```python
from build123d import *

# Parameters (mm, degrees)
BOSS_EXTRUDE1_DEPTH = 6.35
SKETCH2_W           = 25
SKETCH2_H           = 18.64
CUT_EXTRUDE1_DEPTH  = 91.434078201


with BuildPart() as part:
    # Sketch1 → Boss-Extrude1 (new body)
    with BuildSketch(Plane(origin=(0, 0, 0), x_dir=(1, 0, 0), z_dir=(0, 1, 0))):
        with BuildLine():
            Line((7, 0), (70, 0))
            ThreePointArc((70, 0), (74.949747468, 2.050252532), (77, 7))
            Line((77, 7), (77, 40))
            ThreePointArc((77, 40), (74.949747468, 44.949747468), (70, 47))
            Line((70, 47), (7, 47))
            ThreePointArc((7, 47), (2.050252532, 44.949747468), (0, 40))
            Line((0, 40), (0, 7))
            ThreePointArc((0, 7), (2.050252532, 2.050252532), (7, 0))
        make_face()
    extrude(amount=BOSS_EXTRUDE1_DEPTH)

    # Sketch2 → Cut-Extrude1 (cut, through all)
    with BuildSketch(Plane(origin=(0, 6.35, 0), x_dir=(1, 0, 0), z_dir=(0, 1, 0))):
        with Locations((38.5, 16.32)):
            Rectangle(SKETCH2_W, SKETCH2_H)
    extrude(amount=-CUT_EXTRUDE1_DEPTH, mode=Mode.SUBTRACT)


solid = part.part
```
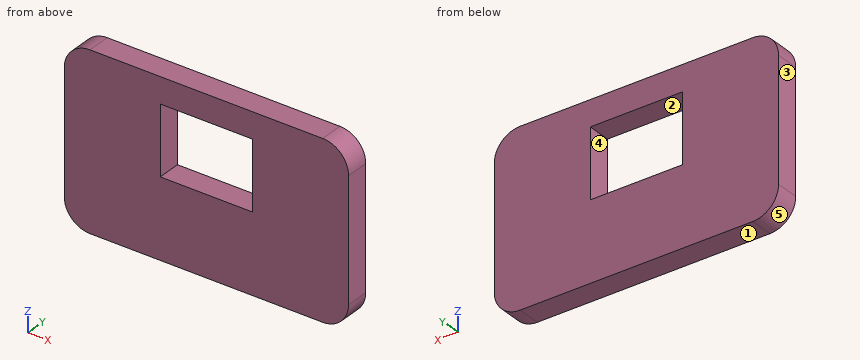
The listing builds one solid part. Answer for the finished solid, in the listing's coordinates (mm). Face numbers are marked on the shaded views. A direction names the side the tool comes from. Give positions to 0.01 mm unless a question says otherwise; leave off trailing zeros. Order: outer loops, then holes, each group sorted by start corner. A loop starts at its lowest first (then second) coordinate and runs counter-clockwise, first axis right, second up. Notation, with made-up numbers: (67, 61.25) - (116, 61.25) arc R12 cw to (116, 78.25) - close; hole circle Ø2 at (37.5, -27). An arc over 180 degrees is marked (long way). Use one line per item in the form item = value. Start each with the question number.
(1) The mould has two halves that part along Z. Classify the marked faces 1, 2 and 3: released by +Z, released by -Z, zero draft, split by the parting line, or undercut.
(2) A cutting plane is placed at A-A, the plane x = 41.5. Write down the section's boundary in (y, z).
(3) A cutting plane is placed at D-D, the plane z = -3.5. Write down the section's boundary in (x, y), then the cut area to 3 significant figures.
(4) A cutting plane is placed at C-C, the plane y = 5. Write down the section's boundary in (x, z), then the cut area to 3 significant figures.
(5) A flat-ended cylindrical pin translates along its axis: pin 1 Ø12 at (x, z) = (33.5, -13.5) entering from +Y. Find the tip coordinate at first contact, or state that the pin passes through.
(6) A cutting plane is placed at B-B, the plane z = -14. Write down the section's boundary in (x, y), then the cut area to 3 significant figures.
(7) For the marked faces 4 and 5, determine the directions among +Z, -Z, +X, -X, +Y, -Y from which every point of the face is accessible in a straight line to the end or side of a thin tool.
(8) Consider line 1 (Z direction, x = 36, y = 5.75); line 2 (X direction, y = 5.25, z = -22.5); line 3 (X direction, y = 5, z = -43). Determine where each line is inside the solid, lowest interval first. Write a range as from..to.
Ans:
q1.face_1 = released by -Z
q1.face_2 = undercut
q1.face_3 = zero draft
q2.outline = (0, -47) - (6.35, -47) - (6.35, -25.64) - (0, -25.64) - close; (0, -7) - (6.35, -7) - (6.35, 0) - (0, 0) - close
q3.outline = (0.94, 0) - (76.06, 0) - (76.06, 6.35) - (0.94, 6.35) - close
q3.area = 477 mm^2
q4.outline = (0, -40) arc R7 ccw to (7, -47) - (70, -47) arc R7 ccw to (77, -40) - (77, -7) arc R7 ccw to (70, 0) - (7, 0) arc R7 ccw to (0, -7) - close; hole (26, -25.64) - (51, -25.64) - (51, -7) - (26, -7) - close
q4.area = 3,110 mm^2
q5.pin_1 = through
q6.outline = (0, 0) - (26, 0) - (26, 6.35) - (0, 6.35) - close; (51, 0) - (77, 0) - (77, 6.35) - (51, 6.35) - close
q6.area = 330 mm^2
q7.face_4 = +Y, -Y
q7.face_5 = -Z, -X, +Y, -Y
q8.line_1 = -47..-25.64, -7..0
q8.line_2 = 0..26, 51..77
q8.line_3 = 0.68..76.32
